Can you work these out from the drawing? Everything is in mm from the part's minimum corner. A direction names the side the tool comes from. Give positions to 0.01 mm unless a question says otherwise; leave off trailing zeros. Write each loop counter-clockwise with the first axis right and the second up, starting at its lowest first coordinate (ties: lowest second). Pieces come first, ordered by that corner, then holes. Notation, with made-up numbers: M 47,-17.5 L 88,-17.5 A18 cw 88,2.5 Z; hole C 42,55 d10. An arc over 180 degrees is marked long. One line per item, written item: value.
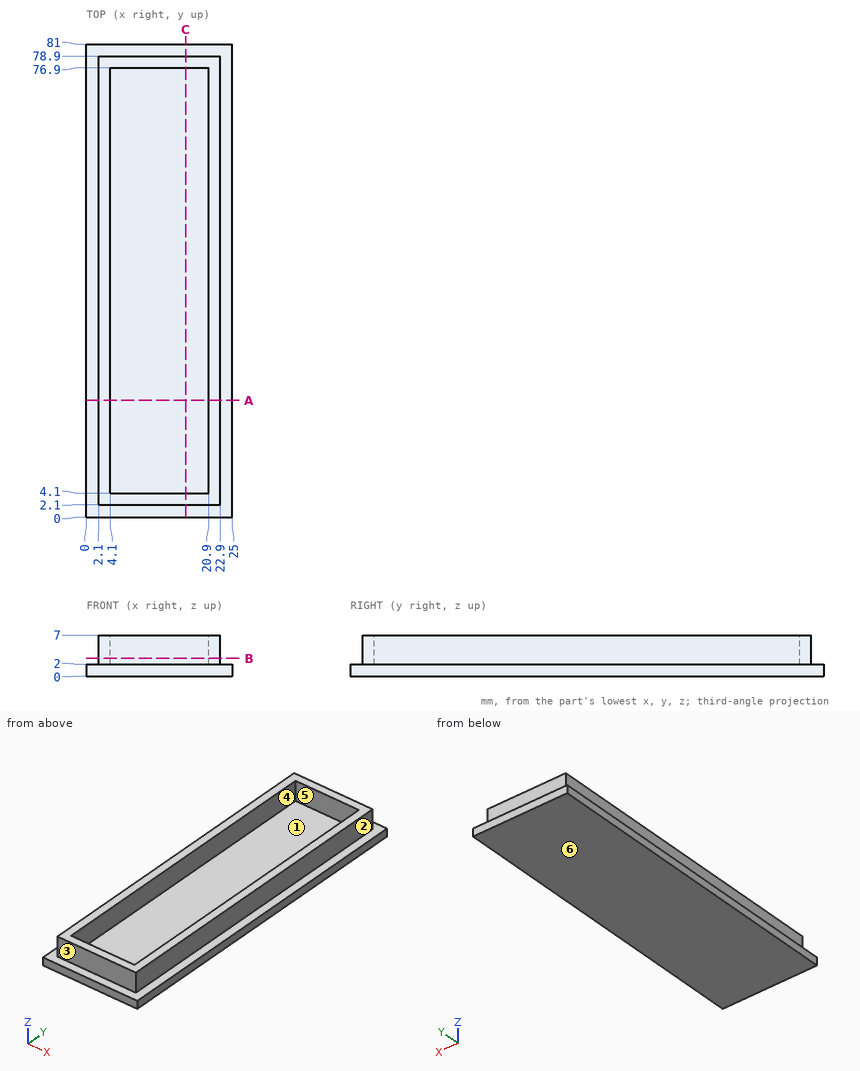
1) If we section it at B-B, the plane z = 3: Write out the boundary of the cut face in (x, y).
Outcome:
outline: M 2.1,2.1 L 22.9,2.1 L 22.9,78.9 L 2.1,78.9 Z; hole M 4.1,4.1 L 20.9,4.1 L 20.9,76.9 L 4.1,76.9 Z
2) We'd pull the mould along Y, two halves only. Please class the marked faces 1, 2, 3 and 4: pulls with the +Y half, pulls with the -Y half, needs draft (parallel to the pull), parting line crosses it, or undercut.
Outcome:
face 1: undercut
face 2: needs draft
face 3: pulls with the -Y half
face 4: undercut
3) On a 3-axis mill with a long thin cutter (end or side, diameter ignored), from which of +Z, -Z, +X, -X, +Y, -Y can I reach the whole of each face in a straight line? I mean the marked faces 5 and 6. Say none if no direction works.
Outcome:
face 5: +Z
face 6: -Z, +X, -X, +Y, -Y
4) I'm going to push flat-ended pins straight in: pin 1 (4 mm diameter, centred on y = 24.5, z = 4.5, fed in from -X); pin 2 (4 mm diameter, centred on x = 16.5, z = 3.5, fed in from -Y); pin 3 (1 mm diameter, centred on x = 18.5, z = 3.5, fed in from -Y); pin 4 (1.5 mm diameter, centred on x = 13.5, z = 4, fed in from +Y). Where does each tip first touch, or does it pass through?
Outcome:
pin 1: stops at x = 2.1
pin 2: stops at y = 0
pin 3: stops at y = 2.1
pin 4: stops at y = 78.9
5) Please list where these lines run through material, in increasing order: L1, parallel to X at y = 30.5, z = 2.5; L2, parallel to Y at x = 18.75, z = 4.25; L3, parallel to Z at x = 8, y = 27. Write a range as from..to.
Outcome:
L1: x = 2.1..4.1, 20.9..22.9
L2: y = 2.1..4.1, 76.9..78.9
L3: z = 0..2
6) If we section it at C-C, the plane x = 17: Write out the boundary of the cut face in (y, z), then the cut area to 3 significant figures.
Outcome:
outline: M 0,0 L 81,0 L 81,2 L 78.9,2 L 78.9,7 L 76.9,7 L 76.9,2 L 4.1,2 L 4.1,7 L 2.1,7 L 2.1,2 L 0,2 Z
area: 182 mm^2
7) If we section it at A-A, the plane y = 20: Write out the boundary of the cut face in (x, z).
Outcome:
outline: M 0,0 L 25,0 L 25,2 L 22.9,2 L 22.9,7 L 20.9,7 L 20.9,2 L 4.1,2 L 4.1,7 L 2.1,7 L 2.1,2 L 0,2 Z
